Here's how the part is built. I have some questions about the finished solid (model axes, mm). Face numbers are marked on the shaded views. A direction names the side the tool comes from. Round coordinates to 2 decimals unless told otherwise and drop trailing zeros. Write each loop counter-clockwise with the first axis right and the second up, starting at its lowest first coordinate (ties: lowest second). Pieces come first, ordered by that corner, then holes. Notation, with made-up numbers: (-33, 59.5) -> (4, 59.5) arc R14 cw to (4, 64.5) -> close; hole circle Ø3 at (66, 80). An arc over 180 degrees is marked (long way). Answer in a Markdown table with one row per item. Add a question column.
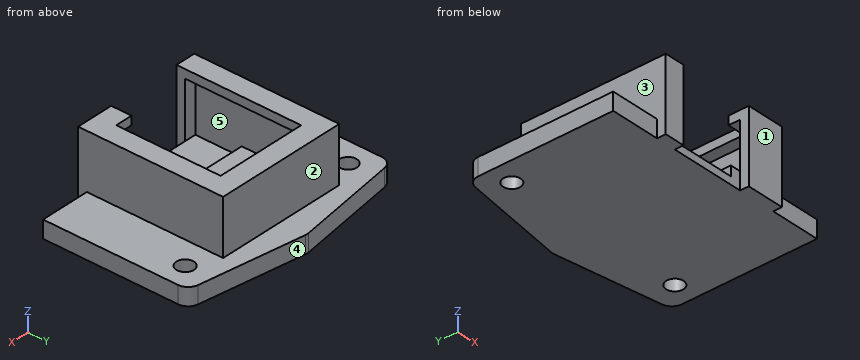
from build123d import *

# Parameters (mm, degrees)
CROQUIS1_R              = 1.5
SALIENTE_EXTRUIR1_DEPTH = 3
SALIENTE_EXTRUIR2_DEPTH = 8
CROQUIS3_W              = 13
CROQUIS3_H              = 1.7
CORTAR_EXTRUIR1_DEPTH   = 8
CROQUIS5_W              = 3.5
CROQUIS5_H              = 11
CROQUIS5_W_2            = 6.5
SALIENTE_EXTRUIR3_DEPTH = 1.5
SALIENTE_EXTRUIR4_DEPTH = 1.5


with BuildPart() as part:
    # Croquis1 → Saliente-Extruir1 (new body)
    with BuildSketch(Plane.XY):
        with BuildLine():
            Line((-55.603283504, 22.637490201), (-73.603283504, 19.937490201))
            ThreePointArc((-73.603283504, 19.937490201), (-74.822083019, 19.26473017), (-75.306602598, 17.959617496))
            Line((-75.306602598, 17.959617496), (-75.306602598, -5.318007663))
            Line((-75.306602598, -5.318007663), (-35.306602598, -5.318007663))
            Line((-35.306602598, -5.318007663), (-35.306602598, 17.959617496))
            ThreePointArc((-35.306602598, 17.959617496), (-35.791122177, 19.26473017), (-37.009921692, 19.937490201))
            Line((-37.009921692, 19.937490201), (-55.009921692, 22.637490201))
            ThreePointArc((-55.009921692, 22.637490201), (-55.306602598, 22.659617496), (-55.603283504, 22.637490201))
        make_face()
        with Locations((-71.306602598, 15.681992337)):
            Circle(CROQUIS1_R, mode=Mode.SUBTRACT)
        with Locations((-39.306602598, 15.681992337)):
            Circle(CROQUIS1_R, mode=Mode.SUBTRACT)
    extrude(amount=SALIENTE_EXTRUIR1_DEPTH)

    # Croquis2 → Saliente-Extruir2 (add)
    with BuildSketch(Plane.XY.offset(3)):
        Polygon((-66.706602598, -5.318007663), (-65.206602598, -5.318007663), (-65.206602598, 16.681992337), (-45.406602598, 16.681992337), (-45.406602598, -5.318007663), (-43.906602598, -5.318007663), (-43.906602598, 18.181992337), (-66.706602598, 18.181992337), align=None)
    extrude(amount=SALIENTE_EXTRUIR2_DEPTH)

    # Croquis3 → Cortar-Extruir1 (cut)
    with BuildSketch(Plane.XZ.offset(5.318007663)):
        with Locations((-58.706602598, 2.15)):
            Rectangle(CROQUIS3_W, CROQUIS3_H)
    extrude(amount=-CORTAR_EXTRUIR1_DEPTH, mode=Mode.SUBTRACT)

    # Croquis5 → Saliente-Extruir3 (add)
    with BuildSketch(Plane.XZ.offset(5.318007663)):
        with Locations((-64.956602598, 5.5)):
            Rectangle(CROQUIS5_W, CROQUIS5_H)
        with Locations((-47.156602598, 5.5)):
            Rectangle(CROQUIS5_W_2, CROQUIS5_H)
    extrude(amount=SALIENTE_EXTRUIR3_DEPTH)

    # Croquis6 → Saliente-Extruir4 (add)
    with BuildSketch(Plane.XY.offset(11)):
        Polygon((-63.206602598, -5.318007663), (-63.206602598, -6.818007663), (-66.706602598, -6.818007663), (-66.706602598, 18.181992337), (-43.906602598, 18.181992337), (-43.906602598, -6.818007663), (-50.406602598, -6.818007663), (-50.406602598, -3.318007663), (-47.406602598, -3.318007663), (-47.406602598, 14.681992337), (-63.206602598, 14.681992337), align=None)
    extrude(amount=SALIENTE_EXTRUIR4_DEPTH)


solid = part.part
Item 1: I need wall thicknesses on line 1 along X through (y, z) = (9.75, 7.25); line 2 along X through (y, z) = (1, 1.5); line 3 along Y through (x, z) = (-65, 5.75). Which ranges of each line are inside material? Lowest first, please. Write a range as from..to.
Item 2: If we section it at A-A on y = -4: Please give me the cut outline in (x, z).
Item 3: For P1, Ø4, axis at x = -48.5, z = 8, coming from the +Y side; P2, Ø3.5, axis at x = -59.5, z = 1, coming from the -Y side; P3, Ø5, axis at y = 3, z = 6.5, coming from the +X side, each with a flat end and sliding along its axis, tell me the tip position at first contact or that it passes through.
Item 4: On a 3-axis mill with a long thin cutter (end or side, diameter ignored), from which of +Z, -Z, +X, -X, +Y, -Y can I reach the whole of each face in a straight line? I mean the marked faces 1 and 2. Say none if no direction works.
Item 5: If we mould it in two halves opening along Y, with no side actions, what happens to the marked faces 3, 4 and 5? For each: pulls with the +Y half, pulls with the -Y half, needs draft (parallel to the pull), parting line crosses it, or undercut.
Item 6: If we section it at C-C on z = 9.5: Please give me the cut outline in (x, y), then the cut area to 3 significant figures.
Item 7: If we section it at D-D on z = 2.5: Please give me the cut outline in (x, y), then the cut area to 3 significant figures.
Item 8: If we section it at B-B on x = -39: Please give me the cut outline in (y, z), then the cut area to 3 significant figures.
Results list:
| question | item | result |
|---|---|---|
| 1 | line 1 | -66.71..-65.21, -45.41..-43.91 |
| 1 | line 2 | -75.31..-65.21, -52.21..-35.31 |
| 1 | line 3 | -6.82..-5.32, 16.68..18.18 |
| 2 | outline | (-75.31, 0) -> (-35.31, 0) -> (-35.31, 3) -> (-43.91, 3) -> (-43.91, 12.5) -> (-50.41, 12.5) -> (-50.41, 11) -> (-45.41, 11) -> (-45.41, 3) -> (-52.21, 3) -> (-52.21, 1.3) -> (-65.21, 1.3) -> (-65.21, 11) -> (-63.21, 11) -> (-63.21, 12.5) -> (-66.71, 12.5) -> (-66.71, 3) -> (-75.31, 3) -> close |
| 3 | P1 | y = 18.18 |
| 3 | P2 | y = -5.32 |
| 3 | P3 | x = -43.91 |
| 4 | face 1 | +Z, -Z, +X, -X, -Y |
| 4 | face 2 | +Z, +X, -X, +Y |
| 5 | face 3 | needs draft |
| 5 | face 4 | pulls with the +Y half |
| 5 | face 5 | undercut |
| 6 | outline | (-66.71, -6.82) -> (-63.21, -6.82) -> (-63.21, -5.32) -> (-65.21, -5.32) -> (-65.21, 16.68) -> (-45.41, 16.68) -> (-45.41, -5.32) -> (-50.41, -5.32) -> (-50.41, -6.82) -> (-43.91, -6.82) -> (-43.91, 18.18) -> (-66.71, 18.18) -> close |
| 6 | area | 115 mm² |
| 7 | outline | (-75.31, -5.32) -> (-66.71, -5.32) -> (-66.71, -6.82) -> (-63.21, -6.82) -> (-63.21, -5.32) -> (-65.21, -5.32) -> (-65.21, 2.68) -> (-52.21, 2.68) -> (-52.21, -5.32) -> (-50.41, -5.32) -> (-50.41, -6.82) -> (-43.91, -6.82) -> (-43.91, -5.32) -> (-35.31, -5.32) -> (-35.31, 17.96) arc R2 ccw to (-37.01, 19.94) -> (-55.01, 22.64) arc R2 ccw to (-55.6, 22.64) -> (-73.6, 19.94) arc R2 ccw to (-75.31, 17.96) -> close; hole circle Ø3 at (-71.31, 15.68); hole circle Ø3 at (-39.31, 15.68) |
| 7 | area | 956 mm² |
| 8 | outline | (-5.32, 0) -> (14.21, 0) -> (14.21, 3) -> (-5.32, 3) -> close; (17.15, 0) -> (20.24, 0) -> (20.24, 3) -> (17.15, 3) -> close |
| 8 | area | 67.9 mm² |
